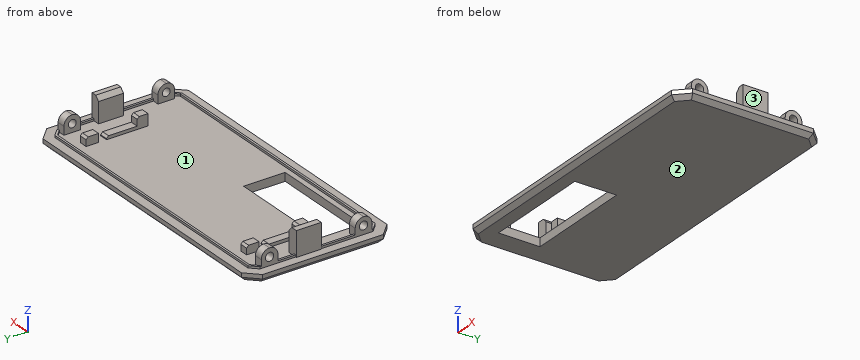
```python
from build123d import *

# Parameters (mm, degrees)
EXTRUDE_1_DEPTH               = 2
CHAMFER_1_SIZE                = 1
SKETCH_3_W                    = 2
SKETCH_3_H                    = 4
EXTRUDE_2_DEPTH               = 4
FILLET_1_R                    = 2
SKETCH_4_R                    = 1
CUT_EXTRUDE_1_DEPTH           = 2
CUT_EXTRUDE_1_DRAFT           = -2
CUT_EXTRUDE_1_PROFILE_2_DEPTH = 2
CUT_EXTRUDE_1_PROFILE_2_DRAFT = -2
SKETCH_5_R                    = 1
CUT_EXTRUDE_2_DEPTH           = 2
CUT_EXTRUDE_2_DRAFT           = -2
CUT_EXTRUDE_2_PROFILE_2_DEPTH = 2
CUT_EXTRUDE_2_PROFILE_2_DRAFT = -2
SKETCH_6_W                    = 2
SKETCH_6_H                    = 10
EXTRUDE_3_DEPTH               = 0.75
SKETCH_7_W                    = 2
SKETCH_7_H                    = 2.6
EXTRUDE_4_DEPTH               = 2
CHAMFER_2_SIZE                = 0.5
SKETCH_8_W                    = 2.55
SKETCH_8_H                    = 6
SKETCH_8_W_2                  = 2.25
EXTRUDE_5_DEPTH               = 6
CHAMFER_3_SIZE                = 1
SKETCH_9_W                    = 2
SKETCH_9_H                    = 3
EXTRUDE_6_DEPTH               = 2
CHAMFER_4_SIZE                = 0.5
CUT_EXTRUDE_3_REACH           = 46.294
SKETCH_10_W                   = 26.2
SKETCH_10_H                   = 10
EXTRUDE_7_DEPTH               = 0.5


with BuildPart() as part:
    # 草图1 → 凸台-拉伸1 (new body)
    with BuildSketch(Plane.XY):
        Polygon((-39.76383505, 14.799206062), (-36.76383505, 17.799206062), (31.23616495, 17.799206062), (34.23616495, 14.799206062), (34.23616495, -14.200793938), (31.23616495, -17.200793938), (-36.76383505, -17.200793938), (-39.76383505, -14.200793938), align=None)
    extrude(amount=EXTRUDE_1_DEPTH)

    # 倒角1
    chamfer_1_edges = [part.edges().sort_by_distance(p)[0] for p in [
        (-38.26383505, -15.700793938, 0),
        (-39.76383505, 0.299206062, 0),
        (-38.26383505, 16.299206062, 0),
        (-2.76383505, 17.799206062, 0),
        (32.73616495, 16.299206062, 0),
        (34.23616495, 0.299206062, 0),
        (32.73616495, -15.700793938, 0),
        (-2.76383505, -17.200793938, 0),
    ]]
    chamfer(chamfer_1_edges, length=CHAMFER_1_SIZE)

    # 草图3 → 凸台-拉伸2 (add)
    with BuildSketch(Plane.XY.offset(2)):
        with Locations((-36.56383505, 11.599206062)):
            Rectangle(SKETCH_3_W, SKETCH_3_H)
        with Locations((-36.56383505, -11.000793938)):
            Rectangle(SKETCH_3_W, SKETCH_3_H)
        with Locations((31.03616495, 11.599206062)):
            Rectangle(SKETCH_3_W, SKETCH_3_H)
        with Locations((31.03616495, -11.000793938)):
            Rectangle(SKETCH_3_W, SKETCH_3_H)
    extrude(amount=EXTRUDE_2_DEPTH)

    # 圆角1
    fillet_1_edges = [part.edges().sort_by_distance(p)[0] for p in [
        (31.03616495, 13.599206062, 6),
        (31.03616495, 9.599206062, 6),
        (31.03616495, -9.000793938, 6),
        (31.03616495, -13.000793938, 6),
        (-36.56383505, -13.000793938, 6),
        (-36.56383505, -9.000793938, 6),
        (-36.56383505, 13.599206062, 6),
        (-36.56383505, 9.599206062, 6),
    ]]
    fillet(fillet_1_edges, radius=FILLET_1_R - 0.0001)  # a hair under: the kernel refuses the full size


with BuildPart() as cut_extrude_1_tool:
    # 草图4 → 切除-拉伸1 (with draft: the straight prism first)
    with BuildSketch(Plane(origin=(32.03616495, 0, 0), x_dir=(0, 0, -1), z_dir=(1, 0, 0))):
        with Locations((-4, 11.599206062)):
            Circle(SKETCH_4_R)
    extrude(amount=-CUT_EXTRUDE_1_DEPTH)
    # 切除-拉伸1: the draft: its side faces are tilted about the plane it starts from
    cut_extrude_1_sides = [cut_extrude_1_tool.faces().sort_by_distance(p)[0] for p in [
        (31.03616495, 11.599206062, 5),
    ]]
    draft(cut_extrude_1_sides, Plane(origin=(32.03616495, 0, 0), x_dir=(0, 0, -1), z_dir=(1, 0, 0)), CUT_EXTRUDE_1_DRAFT)


with BuildPart() as part_1:
    add(part.part)

    # 切除-拉伸1: cut by cut_extrude_1_tool
    add(cut_extrude_1_tool.part, mode=Mode.SUBTRACT)


with BuildPart() as cut_extrude_1_profile_2_tool:
    # 草图4 → 切除-拉伸1 profile 2 (with draft: the straight prism first)
    with BuildSketch(Plane(origin=(32.03616495, 0, 0), x_dir=(0, 0, -1), z_dir=(1, 0, 0))):
        with Locations((-4, -11.000793938)):
            Circle(SKETCH_4_R)
    extrude(amount=-CUT_EXTRUDE_1_PROFILE_2_DEPTH)
    # 切除-拉伸1 profile 2: the draft: its side faces are tilted about the plane it starts from
    cut_extrude_1_profile_2_sides = [cut_extrude_1_profile_2_tool.faces().sort_by_distance(p)[0] for p in [
        (31.03616495, -11.000793938, 5),
    ]]
    draft(cut_extrude_1_profile_2_sides, Plane(origin=(32.03616495, 0, 0), x_dir=(0, 0, -1), z_dir=(1, 0, 0)), CUT_EXTRUDE_1_PROFILE_2_DRAFT)


with BuildPart() as part_2:
    add(part_1.part)

    # 切除-拉伸1 profile 2: cut by cut_extrude_1_profile_2_tool
    add(cut_extrude_1_profile_2_tool.part, mode=Mode.SUBTRACT)


with BuildPart() as cut_extrude_2_tool:
    # 草图5 → 切除-拉伸2 (with draft: the straight prism first)
    with BuildSketch(Plane.ZY.offset(37.56383505)):
        with Locations((4, 11.599206062)):
            Circle(SKETCH_5_R)
    extrude(amount=-CUT_EXTRUDE_2_DEPTH)
    # 切除-拉伸2: the draft: its side faces are tilted about the plane it starts from
    cut_extrude_2_sides = [cut_extrude_2_tool.faces().sort_by_distance(p)[0] for p in [
        (-36.56383505, 11.599206062, 3),
    ]]
    draft(cut_extrude_2_sides, Plane.ZY.offset(37.56383505), CUT_EXTRUDE_2_DRAFT)


with BuildPart() as part_3:
    add(part_2.part)

    # 切除-拉伸2: cut by cut_extrude_2_tool
    add(cut_extrude_2_tool.part, mode=Mode.SUBTRACT)


with BuildPart() as cut_extrude_2_profile_2_tool:
    # 草图5 → 切除-拉伸2 profile 2 (with draft: the straight prism first)
    with BuildSketch(Plane.ZY.offset(37.56383505)):
        with Locations((4, -11.000793938)):
            Circle(SKETCH_5_R)
    extrude(amount=-CUT_EXTRUDE_2_PROFILE_2_DEPTH)
    # 切除-拉伸2 profile 2: the draft: its side faces are tilted about the plane it starts from
    cut_extrude_2_profile_2_sides = [cut_extrude_2_profile_2_tool.faces().sort_by_distance(p)[0] for p in [
        (-36.56383505, -11.000793938, 3),
    ]]
    draft(cut_extrude_2_profile_2_sides, Plane.ZY.offset(37.56383505), CUT_EXTRUDE_2_PROFILE_2_DRAFT)


with BuildPart() as part_4:
    add(part_3.part)

    # 切除-拉伸2 profile 2: cut by cut_extrude_2_profile_2_tool
    add(cut_extrude_2_profile_2_tool.part, mode=Mode.SUBTRACT)

    # 草图6 → 凸台-拉伸3 (add)
    with BuildSketch(Plane.XY.offset(2)):
        with Locations((-30.26383505, 2.799206062)):
            Rectangle(SKETCH_6_W, SKETCH_6_H)
        with Locations((24.73616495, 2.799206062)):
            Rectangle(SKETCH_6_W, SKETCH_6_H)
    extrude(amount=EXTRUDE_3_DEPTH)

    # 草图7 → 凸台-拉伸4 (add)
    with BuildSketch(Plane.XY.offset(2.75)):
        with Locations((-30.26383505, -0.900793938)):
            Rectangle(SKETCH_7_W, SKETCH_7_H)
        with Locations((24.73616495, -0.900793938)):
            Rectangle(SKETCH_7_W, SKETCH_7_H)
    extrude(amount=EXTRUDE_4_DEPTH)

    # 倒角2
    chamfer_2_edges = [part_4.edges().sort_by_distance(p)[0] for p in [
        (-30.26383505, 7.799206062, 2.75),
        (24.73616495, 7.799206062, 2.75),
        (-30.26383505, 0.399206062, 4.75),
        (24.73616495, 0.399206062, 4.75),
    ]]
    chamfer(chamfer_2_edges, length=CHAMFER_2_SIZE)

    # 草图8 → 凸台-拉伸5 (add)
    with BuildSketch(Plane.XY.offset(2)):
        with Locations((-36.48883505, 2.299206062)):
            Rectangle(SKETCH_8_W, SKETCH_8_H)
        with Locations((31.11116495, 2.299206062)):
            Rectangle(SKETCH_8_W_2, SKETCH_8_H)
    extrude(amount=EXTRUDE_5_DEPTH)

    # 倒角3
    chamfer_3_edges = [part_4.edges().sort_by_distance(p)[0] for p in [
        (-35.21383505, 2.299206062, 8),
        (29.98616495, 2.299206062, 8),
    ]]
    chamfer(chamfer_3_edges, length=CHAMFER_3_SIZE)

    # 草图9 → 凸台-拉伸6 (add)
    with BuildSketch(Plane.XY.offset(2)):
        with Locations((-30.26383505, 11.199206062)):
            Rectangle(SKETCH_9_W, SKETCH_9_H)
        with Locations((24.73616495, 11.199206062)):
            Rectangle(SKETCH_9_W, SKETCH_9_H)
    extrude(amount=EXTRUDE_6_DEPTH)

    # 倒角4
    chamfer_4_edges = [part_4.edges().sort_by_distance(p)[0] for p in [
        (-30.26383505, 12.699206062, 4),
        (24.73616495, 12.699206062, 4),
    ]]
    chamfer(chamfer_4_edges, length=CHAMFER_4_SIZE)

    # 草图10 → 切除-拉伸3 (cut, up to next)
    with BuildSketch(Plane(origin=(0, 0, 0), x_dir=(-1, 0, 0), z_dir=(0, 0, -1)), mode=Mode.PRIVATE) as cut_extrude_3_sk1:
        with Locations((20.66383505, -8.200793938)):
            Rectangle(SKETCH_10_W, SKETCH_10_H)
    cut_extrude_3_tool1 = extrude(cut_extrude_3_sk1.sketch, amount=-CUT_EXTRUDE_3_REACH, mode=Mode.PRIVATE) & part_4.part
    add(cut_extrude_3_tool1.solids().sort_by_distance((-20.663835, -8.200794, 0))[0], mode=Mode.SUBTRACT)

    # 草图11 → 凸台-拉伸7 (add)
    with BuildSketch(Plane.XY.offset(2)):
        Polygon((30.324895113, 15.599206062), (-35.852565213, 15.599206062), (-37.56383505, 13.887936224), (-37.56383505, -13.289524101), (-35.852565213, -15.000793938), (30.324895113, -15.000793938), (32.03616495, -13.289524101), (32.03616495, 13.887936224), align=None)
        Polygon((30.117788331, 15.099206062), (-35.645458432, 15.099206062), (-37.06383505, 13.680829443), (-37.06383505, -13.08241732), (-35.645458432, -14.500793938), (30.117788331, -14.500793938), (31.53616495, -13.08241732), (31.53616495, 13.680829443), align=None, mode=Mode.SUBTRACT)
    extrude(amount=EXTRUDE_7_DEPTH)


solid = part_4.part
```
Can you work these out from the model? Positions are in its coordinate system, mm. Face numbers are marked on the shaded views. Round coordinates to 2 decimals unless told otherwise and drop trailing zeros. Loops run counter-clockwise (first coordinate to the right, second up) from the corner with the lowest first, then second, coordinate; pieces in that order, holes last.
Item 1: Will these pins go through, and if not, where does the flat tip stop? pin 1 Ø3 at (y, z) = (-12, 4.5) entering from -X; pin 2 Ø1.6 at (y, z) = (11.5, 3) entering from +X; pin 3 Ø1.8 at (y, z) = (2.5, 3.5) entering from -X.
Item 2: Suppose I cut it at A-A, the plane x = -15.5. Write out the boundary of the cut face in (y, z), then the cut area to 3 significant figures.
Item 3: If we mould it in two halves opening along X, with no side actions, what happens to the marked faces 1, 2 and 3? For each: +X half, -X half, draft (parallel to the pull), parting line (faces both ways), or undercut.
Item 4: Suppose I cut it at B-B, the plane y = 2.5. Write out the boundary of the cut face in (x, z).
Item 5: Please list where these lines run through material, in increasing order: L1, parallel to X at y = 3.5, z = 3.75; L2, parallel to Y at x = -2, z = 2.25; L3, parallel to X at y = -12, z = 5.5.
Item 6: Suppose I cut it at C-C, the plane x = 0. Write out the boundary of the cut face in (y, z).
Reported:
1. pin 1: stops at x = -37.56
1. pin 2: stops at x = 32.04
1. pin 3: stops at x = -37.76
2. outline: (-17.2, 1) - (-16.2, 0) - (-13.2, 0) - (-13.2, 2) - (-14.5, 2) - (-14.5, 2.5) - (-15, 2.5) - (-15, 2) - (-17.2, 2) - close; (-3.2, 0) - (16.8, 0) - (17.8, 1) - (17.8, 2) - (15.6, 2) - (15.6, 2.5) - (15.1, 2.5) - (15.1, 2) - (-3.2, 2) - close
2. area: 49.5 mm2
3. face 1: undercut
3. face 2: draft
3. face 3: +X half
4. outline: (-39.76, 1) - (-38.76, 0) - (33.24, 0) - (34.24, 1) - (34.24, 2) - (32.24, 2) - (32.24, 8) - (30.99, 8) - (29.99, 7) - (29.99, 2) - (25.74, 2) - (25.74, 2.75) - (23.74, 2.75) - (23.74, 2) - (-29.26, 2) - (-29.26, 2.75) - (-31.26, 2.75) - (-31.26, 2) - (-35.21, 2) - (-35.21, 7) - (-36.21, 8) - (-37.76, 8) - (-37.76, 2) - (-39.76, 2) - close
5. L1: x = -37.76 to -35.21, 29.99 to 32.24
5. L2: y = -15 to -14.5, 15.1 to 15.6
5. L3: x = -37.56 to -35.56, 30.04 to 32.04
6. outline: (-17.2, 1) - (-16.2, 0) - (16.8, 0) - (17.8, 1) - (17.8, 2) - (15.6, 2) - (15.6, 2.5) - (15.1, 2.5) - (15.1, 2) - (-14.5, 2) - (-14.5, 2.5) - (-15, 2.5) - (-15, 2) - (-17.2, 2) - close
